The model under review builds one solid part; all positions refer to its coordinate system, in mm. A direction names the side the tool comes from. Round coordinates to 2 decimals unless told otherwise and drop trailing zeros. Write each loop counter-clockwise with the first axis right and the second up, starting at its lowest first coordinate (ties: lowest second). Pieces come first, ordered by that corner, then holes. Notation, with made-up numbers: (37, -30.5) -> (53, -30.5) arc R29 ccw to (53, -1.5) -> close; hole circle Ø5 at (35, 67.5). An arc over 180 degrees is marked (long way). Return JSON: item names as keys, results as strings. Group by question number.
1. Clearance check with flat-ended pins moving along their axes: P1, Ø2, axis at y = -0.5, z = 3, coming from the +X side; P2, Ø2.5, axis at x = 40.13, y = -4.18, coming from the +Z side; P3, Ø14.5, axis at x = 38.5, y = -33.5, coming from the +Z side; P4, Ø2, axis at x = 25, z = 1.5, coming from the +Y side. State where each tip first meets the part, or that it passes through.
2. Take a section at C-C, the plane x = 35.5. Write out the cut boundary in (y, z), then the cut area to 3 significant figures.
3. Take a section at A-A, the plane x = 18.5. Write out the cut boundary in (y, z), then the cut area to 3 significant figures.
4. Tool access review of faces 1 (the cylindrical face through (67.287, -58.189, 2.028)), 2 (the flat face through (56, -13.524, 5)), 3 (the flat face through (94, -13.524, 2)), 4 (the flat face through (56, -5, 4)), 5 (the flat face through (30.277, -1, 2)): name each direction out of +Z, -Z, +X, -X, +Y, -Y from which nothing blocks a thin tool from reaching the whole face with its end or side.
5. For line 1 along X through (y, z) = (-46.5, 0.75); line 2 along X through (y, z) = (-57.5, 3.5); line 3 along X through (y, z) = (-6, 2), list the stretches that pass through material, from the lowest coordinate up. Write a range as from..to.
6. Mouldability with a two-part tool opening along Y and no side actions: class faces 6 (the cylindrical face through (99.78, -25.76, 2.03)), 7 (the flat face through (20, -13.524, 2)), 8 (the flat face through (56, -40, 0)) as pulls with the +Y half, pulls with the -Y half, needs draft (parallel to the pull), parting line crosses it, or undercut.
7. Take a section at B-B, the plane y = -52.5. Write out the cut boundary in (x, z).
8. Take a section at D-D, the plane y = 5.5. Write out the cut boundary in (x, z).
from build123d import *

# Parameters (mm, degrees)
CROQUIS1_W              = 95
CROQUIS1_H              = 95
SALIENTE_EXTRUIR1_DEPTH = 4
CORTAR_EXTRUIR1_DEPTH   = 100
CROQUIS5_W              = 21
CROQUIS5_H              = 31.5
CORTAR_EXTRUIR2_DEPTH   = 100
CROQUIS6_W              = 21
CROQUIS6_H              = 31.5
CORTAR_EXTRUIR3_DEPTH   = 100
CROQUIS7_W              = 3
CROQUIS7_H              = 15
CORTAR_EXTRUIR4_DEPTH   = 100
REDONDEO1_R             = 1
CROQUIS8_R              = 5
CORTAR_EXTRUIR5_DEPTH   = 10
SALIENTE_EXTRUIR2_DEPTH = 53
CROQUIS10_R             = 1.5
CORTAR_EXTRUIR6_DEPTH   = 10
CROQUIS11_R             = 1.45
CORTAR_EXTRUIR7_DEPTH   = 20


with BuildPart() as part:
    # Croquis1 → Saliente-Extruir1 (new body)
    with BuildSketch(Plane.XY):
        with Locations((56.776857567, -29.52358237)):
            Rectangle(CROQUIS1_W, CROQUIS1_H)
    extrude(amount=SALIENTE_EXTRUIR1_DEPTH)

    # Croquis3 → Cortar-Extruir1 (cut)
    with BuildSketch(Plane.ZY.offset(-9.276857567)):
        Polygon((4, -62.076521477), (0, -77.02358237), (4, -77.02358237), align=None)
    extrude(amount=-CORTAR_EXTRUIR1_DEPTH, mode=Mode.SUBTRACT)

    # Croquis5 → Cortar-Extruir2 (cut)
    with BuildSketch(Plane.XY.offset(4)):
        with Locations((19.776857567, 2.22641763)):
            Rectangle(CROQUIS5_W, CROQUIS5_H)
    extrude(amount=-CORTAR_EXTRUIR2_DEPTH, mode=Mode.SUBTRACT)

    # Croquis6 → Cortar-Extruir3 (cut)
    with BuildSketch(Plane.XY.offset(4)):
        with Locations((93.776857567, 2.22641763)):
            Rectangle(CROQUIS6_W, CROQUIS6_H)
    extrude(amount=-CORTAR_EXTRUIR3_DEPTH, mode=Mode.SUBTRACT)

    # Croquis7 → Cortar-Extruir4 (cut)
    with BuildSketch(Plane.ZY.offset(-30.276857567)):
        with Locations((3.808437884, 5.867431485)):
            Rectangle(CROQUIS7_W, CROQUIS7_H)
    extrude(amount=-CORTAR_EXTRUIR4_DEPTH, mode=Mode.SUBTRACT)

    # Redondeo1
    redondeo1_edges = [part.edges().sort_by_distance(p)[0] for p in [
        (56.776857567, 17.97641763, 0),
    ]]
    fillet(redondeo1_edges, radius=REDONDEO1_R)

    # Croquis8 → Cortar-Extruir5 (cut)
    with BuildSketch(Plane(origin=(0, 0, 0), x_dir=(-1, 0, 0), z_dir=(0, 0, -1))):
        with Locations((-93.276857567, -54.130923869)):
            Circle(CROQUIS8_R)
        with Locations((-20.276857567, -54.130923869)):
            Circle(CROQUIS8_R)
    extrude(amount=-CORTAR_EXTRUIR5_DEPTH, mode=Mode.SUBTRACT)

    # Croquis9 → Saliente-Extruir2 (add)
    with BuildSketch(Plane.ZY.offset(-30.276857567)):
        Polygon((4, -13.52358237), (4, -8.52358237), (6.2, -13.52358237), align=None)
    extrude(amount=-SALIENTE_EXTRUIR2_DEPTH)

    # Croquis10 → Cortar-Extruir6 (cut)
    with BuildSketch(Plane.XY.offset(4)):
        with Locations((12.276857567, -25.82358237)):
            Circle(CROQUIS10_R)
        with Locations((12.276857567, -46.52358237)):
            Circle(CROQUIS10_R)
        with Locations((45.076857567, -57.276521477)):
            Circle(CROQUIS10_R)
        with Locations((68.476857567, -57.276521477)):
            Circle(CROQUIS10_R)
        with Locations((101.276857567, -25.82358237)):
            Circle(CROQUIS10_R)
        with Locations((101.276857567, -46.52358237)):
            Circle(CROQUIS10_R)
    extrude(amount=-CORTAR_EXTRUIR6_DEPTH, mode=Mode.SUBTRACT)

    # Croquis11 → Cortar-Extruir7 (cut)
    with BuildSketch(Plane.XY.offset(4)):
        with Locations((40.129677313, 15.935254897)):
            Circle(CROQUIS11_R)
        with Locations((73.424037821, 15.935254897)):
            Circle(CROQUIS11_R)
        with Locations((40.129677313, -4.182419638)):
            Circle(CROQUIS11_R)
        with Locations((73.424037821, -4.182419638)):
            Circle(CROQUIS11_R)
    extrude(amount=-CORTAR_EXTRUIR7_DEPTH, mode=Mode.SUBTRACT)


solid = part.part
Output:
{
 "1": {"P1": "stops at x = 83.28", "P2": "passes through", "P3": "stops at z = 4", "P4": "stops at y = -13.52"},
 "2": {"outline": "(-77.02, 0) -> (16.98, 0) arc R1 ccw to (17.98, 1) -> (17.98, 4) -> (13.37, 4) -> (13.37, 2.31) -> (-1.63, 2.31) -> (-1.63, 4) -> (-8.52, 4) -> (-13.52, 6.2) -> (-13.52, 4) -> (-62.08, 4) -> close", "area": "330 mm^2"},
 "3": {"outline": "(-77.02, 0) -> (-58.8, 0) -> (-58.8, 4) -> (-62.08, 4) -> close; (-49.46, 0) -> (-13.52, 0) -> (-13.52, 4) -> (-49.46, 4) -> close", "area": "187 mm^2"},
 "4": {"face 1": "+Z, -Z", "face 2": "+Z, +X, -X, -Y", "face 3": "+Z, -Z, +X, +Y", "face 4": "+Z, +X, -X, +Y", "face 5": "+Z, -Z, -X, +Y"},
 "5": {"line 1": "x = 9.28..10.78, 13.78..99.78, 102.78..104.28", "line 2": "x = 9.28..16.58, 23.97..43.59, 46.56..66.99, 69.96..89.58, 96.97..104.28", "line 3": "x = 30.28..83.28"},
 "6": {"face 6": "undercut", "face 7": "pulls with the +Y half", "face 8": "needs draft"},
 "7": {"outline": "(9.28, 0) -> (15.55, 0) -> (15.55, 4) -> (9.28, 4) -> close; (25, 0) -> (88.55, 0) -> (88.55, 4) -> (25, 4) -> close; (98, 0) -> (104.28, 0) -> (104.28, 4) -> (98, 4) -> close"},
 "8": {"outline": "(30.28, 0) -> (83.28, 0) -> (83.28, 2.31) -> (30.28, 2.31) -> close"}
}
